Geometry check sheet. Reference: the model listing, model coordinates, mm. Give positions to 0.01 mm unless a question says otherwise; leave off trailing zeros. Loops run counter-clockwise (first coordinate to the right, second up) from the corner with the lowest first, then second, coordinate; pieces in that order, holes last. Notation, with made-up numbers: (73.5, 73) - (123.5, 73) arc R34 cw to (123.5, 108) - close; hole circle Ø7 at (6.5, 81). An arc over 180 degrees is marked (long way). Write item = value, one per line. Start each with the question number.
Autodesk Fusion 360 part; units mm, degrees
sketch "Sketch1" plane through (0, 0, 0) normal (0, 0, 1) x (1, 0, 0)
  line L0 (0, 0) -> (0, 25)
  line L1 (0, 25) -> (200, 25)
  line L2 (200, 25) -> (200, 0)
  line L3 (200, 0) -> (0, 0)
  line L4 (0, 12.5) -> (15, 12.5)
  circle A0 centre (15, 12.5) radius 5
  dimension "d2" = 200
  dimension "d3" = 25
extrude "Extrude1" add sketch "Sketch1" along normal blind 1
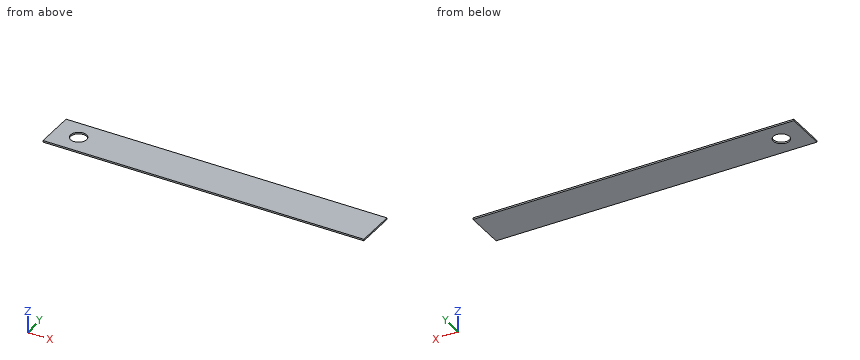
1) Cross-section at B-B on y = 12.5. Enter the section's corners in (x, z).
2) Cross-section at C-C on z = 0.5. Enter the section's corners in (x, y).
3) Material ranges on line 1 along Y through (x, z) = (15, 0.45); line 2 along X through (y, z) = (12.5, 0.8); line 3 along Y through (x, z) = (18, 0.6), recorded low to high.
4) Cross-section at A-A on x = 15. Enter the section's corners in (y, z).
Checked values:
q1.outline = (0, 0) - (10, 0) - (10, 1) - (0, 1) - close; (20, 0) - (200, 0) - (200, 1) - (20, 1) - close
q2.outline = (0, 0) - (200, 0) - (200, 25) - (0, 25) - close; hole circle Ø10 at (15, 12.5)
q3.line_1 = 0 to 7.5, 17.5 to 25
q3.line_2 = 0 to 10, 20 to 200
q3.line_3 = 0 to 8.5, 16.5 to 25
q4.outline = (0, 0) - (7.5, 0) - (7.5, 1) - (0, 1) - close; (17.5, 0) - (25, 0) - (25, 1) - (17.5, 1) - close
